Part model, mm, in its own coordinate system. A direction names the side the tool comes from. Give positions to 0.01 mm unless a question says otherwise; leave off trailing zeros. Write item = value, one per line. Start each with the question number.
(1) Which spindle directions (+Z, -Z, +X, -X, +Y, -Y) get a long thin tool onto all of the face, cutting with end or side? Do faces 1 (the flat face through (-70, 15.24, 1)), 2 (the conical face through (-130.612, 46.742, -5.609)), 3 (the flat face through (-60, 10, 26.366)), 4 (the flat face through (-57.8, -26.2, -2.209)), 5 (the flat face through (-57.8, 26.2, 10.491)). Say none if no direction does.
(2) Two-plate mould, pull along Y, no slides. Class faces 6 (the flat face through (-79, 10, -24.434)), 7 (the conical face through (1.471, 29.489, 7.605)), 8 (the cylindrical face through (-70.17, -12.69, 1.32)): pulls with the +Y half, pulls with the -Y half, needs draft (parallel to the pull), parting line crosses it, or undercut.
(3) Probe line 1 along X through (y, z) = (0, -14.5); line 2 along X through (y, z) = (47, -4.5); line 3 along Z through (x, y) = (-126, 47). List the from-to ranges inside material, lowest first. Write a range as from..to.
(4) Flat gauge pins, fed straight in: pin 1 (5 mm diameter, centred on x = -56.5, z = 4, fed in from +Y); pin 2 (3 mm diameter, centred on x = -35, y = 44, fed in from -Z); pin 3 (6 mm diameter, centred on x = -83, z = 1.5, fed in from -Y). Where does each tip first touch, or does it go through?
from build123d import *

# Parameters (mm, degrees)
F3_DEPTH = 50.801
F2_R     = 63.5
F2_R_2   = 22.225
F4_DEPTH = 15.875
F5_R     = 63.5
F5_R_2   = 22.225
F6_DEPTH = 15.875
F7_R     = 6.35


with BuildPart() as f1:
    # F0 (on Front) → F1 (revolve)
    with BuildSketch(Plane.XZ):
        Polygon((-69.6527920461, 26.3657749056), (-69.6527920461, -24.4342250944), (-47.4277920461, -24.4342250944), (-47.4277920461, -18.0842250944), (19.2472079539, -18.0842250944), (19.2472079539, -10.0066470696), (6.5472079539, -5.3842250944), (6.5472079539, 7.3157749056), (19.2472079539, 11.9381968808), (19.2472079539, 20.0157749056), (-47.4277920461, 20.0157749056), (-47.4277920461, 26.3657749056), align=None)
    revolve(axis=Axis((-69.6527920461, 0, 0.9657749056), (0, 0, -1)))

    # F2 (on face) → F3 (cut, through all)
    with BuildSketch(Plane.XY.offset(26.3657749056)):
        with BuildLine():
            Line((-72.8277920461, 15.24), (-72.8277920461, 12.2967221242))
            ThreePointArc((-72.8277920461, 12.2967221242), (-69.6527920461, -12.7), (-66.4777920461, 12.2967221242))
            Line((-66.4777920461, 12.2967221242), (-66.4777920461, 15.24))
            Line((-66.4777920461, 15.24), (-72.8277920461, 15.24))
        make_face()
    extrude(amount=-F3_DEPTH, mode=Mode.SUBTRACT)

    # F2 (on face) → F4 (cut)
    with BuildSketch(Plane.XY.offset(26.3657749056)):
        with Locations((-69.6527920461, 0)):
            Circle(F2_R)
        with Locations((-69.6527920461, 0)):
            Circle(F2_R_2, mode=Mode.SUBTRACT)
    extrude(amount=-F4_DEPTH, mode=Mode.SUBTRACT)

    # F5 (on face) → F6 (cut)
    with BuildSketch(Plane(origin=(0, 0, -18.0842250944), x_dir=(1, 0, 0), z_dir=(0, 0, -1))):
        with Locations((-69.6527920461, 0)):
            Circle(F5_R)
        with Locations((-69.6527920461, 0)):
            Circle(F5_R_2, mode=Mode.SUBTRACT)
    extrude(amount=-F6_DEPTH, mode=Mode.SUBTRACT)

    # F7
    f7_edges = [f1.edges().sort_by_distance(p)[0] for p in [
        (-133.152792, 0, 10.490775),
        (-91.877792, 0, 10.490775),
        (-133.152792, 0, -2.209225),
        (-91.877792, 0, -2.209225),
    ]]
    fillet(f7_edges, radius=F7_R)


solid = f1.part
Results list:
q1.face_1 = +Z, -Z
q1.face_2 = none
q1.face_3 = +Z, +X, -X, +Y, -Y
q1.face_4 = -Z
q1.face_5 = +Z
q2.face_6 = needs draft
q2.face_7 = parting line crosses it
q2.face_8 = undercut
q3.line_1 = -158.55..-133.15, -91.88..-82.35, -56.95..-47.43, -6.15..19.25
q3.line_2 = -129.63..-110.14, -29.17..-9.67
q3.line_3 = -18.08..20.02
q4.pin_1 = 75.45
q4.pin_2 = -2.22
q4.pin_3 = -75.49
